```python
from build123d import *

# Parameters (mm, degrees)
SKETCH1_R           = 2.5
BOSS_EXTRUDE1_DEPTH = 220
FILLET1_R           = 1
FILLET2_R           = 0.5
FILLET3_R           = 0.5
FILLET4_R           = 0.5
FILLET5_R           = 0.5


with BuildPart() as part:
    # Sketch1 → Boss-Extrude1 (new body)
    with BuildSketch(Plane.XY):
        Polygon((13.2, 0), (13.2, 1.8), (15.45, 1.8), (15.45, 3.6), (12.95, 6.1), (7.05, 6.1), (4.55, 3.6), (4.55, 1.8), (6.8, 1.8), (6.8, 0), (0, 0), (0, 6.8), (1.8, 6.8), (1.8, 4.55), (3.6, 4.55), (6.1, 7.05), (6.1, 12.95), (3.6, 15.45), (1.8, 15.45), (1.8, 13.2), (0, 13.2), (0, 20), (6.8, 20), (6.8, 18.2), (4.55, 18.2), (4.55, 16.4), (7.05, 13.9), (12.95, 13.9), (15.45, 16.4), (15.45, 18.2), (13.2, 18.2), (13.2, 20), (20, 20), (20, 13.2), (18.2, 13.2), (18.2, 15.45), (16.4, 15.45), (13.9, 12.95), (13.9, 7.05), (16.4, 4.55), (18.2, 4.55), (18.2, 6.8), (20, 6.8), (20, 0), align=None)
        with Locations((10, 10)):
            Circle(SKETCH1_R, mode=Mode.SUBTRACT)
    extrude(amount=BOSS_EXTRUDE1_DEPTH)

    # Fillet1
    fillet1_edges = [part.edges().sort_by_distance(p)[0] for p in [
        (0, 0, 110),
        (0, 20, 110),
        (20, 20, 110),
        (20, 0, 110),
    ]]
    fillet(fillet1_edges, radius=FILLET1_R)

    # Fillet2
    fillet2_edges = [part.edges().sort_by_distance(p)[0] for p in [
        (4.55, 18.2, 110),
        (4.55, 16.4, 110),
        (7.05, 13.9, 110),
        (12.95, 13.9, 110),
        (15.45, 16.4, 110),
        (15.45, 18.2, 110),
    ]]
    fillet(fillet2_edges, radius=FILLET2_R)

    # Fillet3
    fillet3_edges = [part.edges().sort_by_distance(p)[0] for p in [
        (18.2, 15.45, 110),
        (16.4, 15.45, 110),
        (13.9, 12.95, 110),
        (13.9, 7.05, 110),
        (16.4, 4.55, 110),
        (18.2, 4.55, 110),
    ]]
    fillet(fillet3_edges, radius=FILLET3_R)

    # Fillet4
    fillet4_edges = [part.edges().sort_by_distance(p)[0] for p in [
        (1.8, 4.55, 110),
        (3.6, 4.55, 110),
        (6.1, 7.05, 110),
        (6.1, 12.95, 110),
        (3.6, 15.45, 110),
        (1.8, 15.45, 110),
    ]]
    fillet(fillet4_edges, radius=FILLET4_R)

    # Fillet5
    fillet5_edges = [part.edges().sort_by_distance(p)[0] for p in [
        (15.45, 1.8, 110),
        (15.45, 3.6, 110),
        (12.95, 6.1, 110),
        (7.05, 6.1, 110),
        (4.55, 3.6, 110),
        (4.55, 1.8, 110),
    ]]
    fillet(fillet5_edges, radius=FILLET5_R)


solid = part.part
```
The listing builds one solid part. Answer for the finished solid, in the listing's coordinates (mm). A direction names the side the tool comes from. Coordinates: 2 decimals unless noted, no trailing zeros. Write each loop counter-clockwise with the first axis right and the second up, starting at its lowest first coordinate (ties: lowest second). Pieces come first, ordered by that corner, then holes. Notation, with made-up numbers: M -12.5,80.25 L 27.5,80.25 A32 ccw 27.5,110.25 Z; hole C 61,8 d7. An arc over 180 degrees is marked long. Use a Markdown table: item, result. Add a question column.
1. Which of the six approach directions +Z, -Z, +X, -X, +Y, -Y give full straight-line access (tool end or side, diameter ignored) to faces 4 (the flat face through (10, 6.1, 108)), 5 (the flat face through (10, 13.9, 108)), 6 (the flat face through (6.1, 10, 108))?
2. Given P1, Ø1, axis at x = 8.5, y = 16, coming from the +Z side; P2, Ø0.5, axis at x = 0.5, z = 124, coming from the -Y side; P3, Ø0.5, axis at x = 0.5, z = 108.5, coming from the +Y side, each flat-ended and moving along its own axis, determine where each tip first touches the part or whether it passes through.
3. For a pull along X with two mould halves and no side action, classify faces 1 (the flat face through (0, 16, 108)), 2 (the flat face through (16, 0, 108)), 3 (the cylindrical face through (9.46, 7.56, 108.46)) as +X half, -X half, draft (parallel to the pull), parting line (faces both ways), or undercut.
4. Straight lines are drawn through the part: line 1 along X through (y, z) = (16.75, 57); line 2 along Y through (x, z) = (10, 62); line 3 along X through (y, z) = (6, 136). For each, find the intervals that lie inside material, in ascending order. Write a range as [from, to].
5. Section A-A (y = 10) is taken. Give the vertices of the cut face in (x, z).
Data:
| question | item | result |
|---|---|---|
| 1 | face 4 | +Z, -Z, -Y |
| 1 | face 5 | +Z, -Z, +Y |
| 1 | face 6 | +Z, -Z, -X |
| 2 | P1 | passes through |
| 2 | P2 | stops at y = 0.03 |
| 2 | P3 | stops at y = 19.97 |
| 3 | face 1 | -X half |
| 3 | face 2 | draft |
| 3 | face 3 | undercut |
| 4 | line 1 | x = [0, 4.55], [15.45, 20] |
| 4 | line 2 | y = [6.1, 7.5], [12.5, 13.9] |
| 4 | line 3 | x = [0, 1.8], [5.05, 6.96], [13.04, 14.95], [18.2, 20] |
| 5 | outline | M 6.1,0 L 7.5,0 L 7.5,220 L 6.1,220 Z; M 12.5,0 L 13.9,0 L 13.9,220 L 12.5,220 Z |
